from build123d import *

# Parameters (mm, degrees)
SKETCH1_W           = 95
SKETCH1_H           = 60
BOSS_EXTRUDE1_DEPTH = 6
SKETCH6_R           = 3.5
SKETCH6_R_2         = 1.5
CUT_EXTRUDE3_DEPTH  = 113.521109131
CUT_EXTRUDE1_DEPTH  = 113.521109131
FILLET3_R           = 1.5
SKETCH7_W           = 8.5
SKETCH7_H           = 3
SKETCH7_H_2         = 7
CUT_EXTRUDE4_DEPTH  = 113.521109131
FILLET4_R           = 5
FILLET5_R           = 1.5
BOSS_EXTRUDE2_DEPTH = 1.6
SKETCH10_W          = 102.175429208
SKETCH10_H          = 24.243237214
CUT_EXTRUDE6_DEPTH  = 113.617760589


with BuildPart() as part:
    # Sketch1 → Boss-Extrude1 (new body)
    with BuildSketch(Plane(origin=(0, 0, 0), x_dir=(1, 0, 0), z_dir=(0, 1, 0))):
        with Locations((47.5, 30)):
            Rectangle(SKETCH1_W, SKETCH1_H)
    extrude(amount=BOSS_EXTRUDE1_DEPTH)

    # Sketch6 → Cut-Extrude3 (cut, through all)
    with BuildSketch(Plane.XZ):
        with Locations(Location((86.5, -30, 0), (0, 0, 270))):
            Circle(SKETCH6_R)
        with Locations(Location((8.5, -30, 0), (0, 0, 270))):
            Circle(SKETCH6_R_2)
    extrude(amount=-CUT_EXTRUDE3_DEPTH, mode=Mode.SUBTRACT)

    # Sketch2 → Cut-Extrude1 (cut, through all)
    with BuildSketch(Plane(origin=(0, 6, 0), x_dir=(-1, 0, 0), z_dir=(0, 1, 0))):
        with BuildLine():
            Line((-8.5, -36.5), (-5, -36.5))
            Line((-5, -36.5), (-5, -55))
            Line((-5, -55), (-90, -55))
            Line((-90, -55), (-90, -38.5))
            Line((-90, -38.5), (-86.5, -38.5))
            ThreePointArc((-86.5, -38.5), (-78, -30), (-86.5, -21.5))
            Line((-86.5, -21.5), (-90, -21.5))
            Line((-90, -21.5), (-90, -5))
            Line((-90, -5), (-5, -5))
            Line((-5, -5), (-5, -23.5))
            Line((-5, -23.5), (-8.5, -23.5))
            ThreePointArc((-8.5, -23.5), (-15, -30), (-8.5, -36.5))
        make_face()
    extrude(amount=-CUT_EXTRUDE1_DEPTH, mode=Mode.SUBTRACT)

    # Fillet3
    fillet3_edges = [part.edges().sort_by_distance(p)[0] for p in [
        (90, 3, -55),
    ]]
    fillet(fillet3_edges, radius=FILLET3_R)

    # Sketch7 → Cut-Extrude4 (cut, through all)
    with BuildSketch(Plane(origin=(0, 6, 0), x_dir=(-1, 0, 0), z_dir=(0, 1, 0))):
        with Locations((-4.25, -30)):
            Rectangle(SKETCH7_W, SKETCH7_H)
        with Locations((-90.75, -30)):
            Rectangle(SKETCH7_W, SKETCH7_H_2)
    extrude(amount=-CUT_EXTRUDE4_DEPTH, mode=Mode.SUBTRACT)

    # Fillet4
    fillet4_edges = [part.edges().sort_by_distance(p)[0] for p in [
        (0, 3, -60),
        (95, 3, -60),
        (0, 3, -28.5),
        (95, 3, 0),
        (0, 3, -31.5),
        (0, 3, 0),
        (95, 3, -33.5),
        (95, 3, -26.5),
    ]]
    fillet(fillet4_edges, radius=FILLET4_R)

    # Fillet5
    fillet5_edges = [part.edges().sort_by_distance(p)[0] for p in [
        (5, 3, -5),
        (5, 3, -23.5),
        (5, 3, -36.5),
        (5, 3, -55),
        (90, 3, -38.5),
        (90, 3, -21.5),
        (90, 3, -5),
    ]]
    fillet(fillet5_edges, radius=FILLET5_R)

    # Sketch9 → Boss-Extrude2 (add)
    with BuildSketch(Plane(origin=(0, 6, 0), x_dir=(1, 0, 0), z_dir=(0, 1, 0))):
        with BuildLine():
            Line((6.5, 4.2), (88.5, 4.2))
            ThreePointArc((88.5, 4.2), (90.126345597, 4.873654403), (90.8, 6.5))
            Line((90.8, 6.5), (90.8, 20))
            ThreePointArc((90.8, 20), (90.126345597, 21.626345597), (88.5, 22.3))
            Line((88.5, 22.3), (86.5, 22.3))
            ThreePointArc((86.5, 22.3), (78.8, 30), (86.5, 37.7))
            Line((86.5, 37.7), (88.5, 37.7))
            ThreePointArc((88.5, 37.7), (90.126345597, 38.373654403), (90.8, 40))
            Line((90.8, 40), (90.8, 53.5))
            ThreePointArc((90.8, 53.5), (90.126345597, 55.126345597), (88.5, 55.8))
            Line((88.5, 55.8), (6.5, 55.8))
            ThreePointArc((6.5, 55.8), (4.873654403, 55.126345597), (4.2, 53.5))
            Line((4.2, 53.5), (4.2, 38))
            ThreePointArc((4.2, 38), (4.873654403, 36.373654403), (6.5, 35.7))
            Line((6.5, 35.7), (8.5, 35.7))
            ThreePointArc((8.5, 35.7), (14.2, 30), (8.5, 24.3))
            Line((8.5, 24.3), (6.5, 24.3))
            ThreePointArc((6.5, 24.3), (4.873654403, 23.626345597), (4.2, 22))
            Line((4.2, 22), (4.2, 6.5))
            ThreePointArc((4.2, 6.5), (4.873654403, 4.873654403), (6.5, 4.2))
        make_face()
    extrude(amount=BOSS_EXTRUDE2_DEPTH)

    # Sketch10 → Cut-Extrude6 (cut, through all)
    with BuildSketch(Plane.XY):
        with Locations((51.087714604, -6.121618607)):
            Rectangle(SKETCH10_W, SKETCH10_H)
    extrude(amount=-CUT_EXTRUDE6_DEPTH, mode=Mode.SUBTRACT)


solid = part.part
Can you work these out from the model? Positions are in its coordinate system, mm. A direction names the side the tool comes from. Coordinates: 2 decimals unless noted, no trailing zeros. Loops run counter-clockwise (first coordinate to the right, second up) from the corner with the lowest first, then second, coordinate; pieces in that order, holes last. Notation, with made-up numbers: (9.25, 81) - (54.25, 81) arc R7 ccw to (54.25, 91) - close; hole circle Ø10 at (89, 89.5). An arc over 180 degrees is marked (long way). Put each result on its own line as item: value. Start each with the question number.
Item 1: Suppose I cut it at A-A (y = 7.05). Please give me the cut outline in (x, z), and give its area (3 significant figures).
Item 2: Which directions (+Z, -Z, +X, -X, +Y, -Y) give clear straight access to the entire face, cutting with the end or side of a thin tool? Please do faces 1 (the face through (47, 7.6, -30)), 2 (the face through (90.14, 6.79, -21.61)), 3 (the face through (7, 7, -35.7)).
Item 3: If I drill on line 1 along Z through (x, y) = (86.5, 6.6); line 2 along Z through (x, y) = (80.5, 6.35); line 3 along X through (y, z) = (7.3, -33), over which ranges is the centre line in solid material (lowest first)?
Item 4: Suppose I cut it at B-B (z = -30). Please give me the cut outline in (x, y), and give its area (3 significant figures).
Here are the results:
1. outline: (4.2, -53.5) arc R2.3 ccw to (6.5, -55.8) - (88.5, -55.8) arc R2.3 ccw to (90.8, -53.5) - (90.8, -40) arc R2.3 ccw to (88.5, -37.7) - (86.5, -37.7) arc R7.7 cw to (86.5, -22.3) - (88.5, -22.3) arc R2.3 ccw to (90.8, -20) - (90.8, -6.5) arc R2.3 ccw to (88.5, -4.2) - (6.5, -4.2) arc R2.3 ccw to (4.2, -6.5) - (4.2, -22) arc R2.3 ccw to (6.5, -24.3) - (8.5, -24.3) arc R5.7 cw to (8.5, -35.7) - (6.5, -35.7) arc R2.3 ccw to (4.2, -38) - close
1. area: 4,200 mm²
2. face 1: +Z, -Z, +X, -X, +Y
2. face 2: +X, +Y, -Y
2. face 3: -X, +Y, -Y
3. line 1: -55.8 to -37.7, -22.3 to -4.2
3. line 2: -55.8 to -34.83, -25.17 to -4.2
3. line 3: 13.35 to 79.41
4. outline: (14.2, 6) - (78.8, 6) - (78.8, 7.6) - (14.2, 7.6) - close
4. area: 103 mm²
